Design review of the part built by this model. Coordinates are the model's own, in mm. Coordinates: 2 decimals unless noted, no trailing zeros. Loops run counter-clockwise (first coordinate to the right, second up) from the corner with the lowest first, then second, coordinate; pieces in that order, holes last. Notation, with made-up numbers: (87.25, -15) -> (105.25, -15) arc R27 cw to (105.25, 1) -> close; hole circle Ø1 at (15, 83). An arc over 180 degrees is marked (long way). Answer as a JSON object with one key per item and string values.
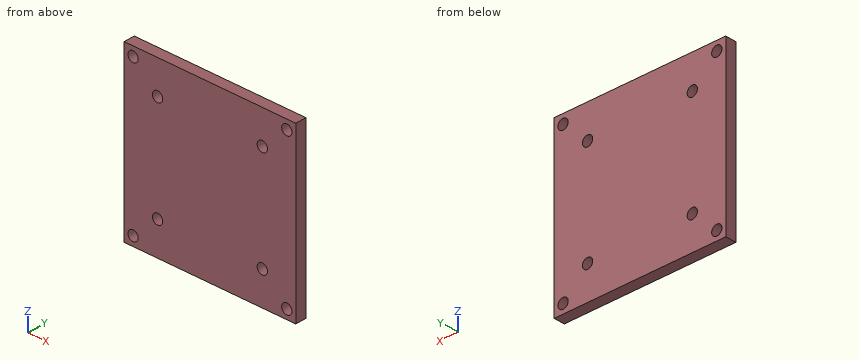
```python
from build123d import *

# Parameters (mm, degrees)
SKETCH1_W           = 50
SKETCH1_H           = 50
SKETCH1_R           = 1.5
BOSS_EXTRUDE1_DEPTH = 3.175


with BuildPart() as part:
    # Sketch1 → Boss-Extrude1 (new body)
    with BuildSketch(Plane(origin=(0, 0, 0), x_dir=(1, 0, 0), z_dir=(0, 1, 0))):
        Rectangle(SKETCH1_W, SKETCH1_H)
        with Locations((-22.4, 22.3)):
            Circle(SKETCH1_R, mode=Mode.SUBTRACT)
        with Locations((22.4, 22.3)):
            Circle(SKETCH1_R, mode=Mode.SUBTRACT)
        with Locations((22.4, -22.3)):
            Circle(SKETCH1_R, mode=Mode.SUBTRACT)
        with Locations((-22.4, -22.3)):
            Circle(SKETCH1_R, mode=Mode.SUBTRACT)
        with Locations((-15.25, 15.25)):
            Circle(SKETCH1_R, mode=Mode.SUBTRACT)
        with Locations((15.25, 15.25)):
            Circle(SKETCH1_R, mode=Mode.SUBTRACT)
        with Locations((15.25, -15.25)):
            Circle(SKETCH1_R, mode=Mode.SUBTRACT)
        with Locations((-15.25, -15.25)):
            Circle(SKETCH1_R, mode=Mode.SUBTRACT)
    extrude(amount=BOSS_EXTRUDE1_DEPTH)


solid = part.part
```
1) Add section A-A, the plane x = -22.4. Give the boundary of the cut face in (y, z) (3 decimals), and give its area (3 significant figures).
Completed:
{"outline": "(0, -25) -> (3.175, -25) -> (3.175, -23.8) -> (0, -23.8) -> close; (0, -20.8) -> (3.175, -20.8) -> (3.175, 20.8) -> (0, 20.8) -> close; (0, 23.8) -> (3.175, 23.8) -> (3.175, 25) -> (0, 25) -> close", "area": "140 mm²"}
2) Clearance check with flat-ended pins moving along their axes: pin 1 Ø5 at (x, z) = (22.4, 22.3) entering from +Y (3 decimals); pin 2 Ø2.5 at (x, z) = (22.4, -22.3) entering from +Y. State where each tip first meets the part, or that it passes through.
Completed:
{"pin 1": "y = 3.175", "pin 2": "through"}
3) Add section C-C, the plane z = -15.25. Give the boundary of the cut face in (x, y) (3 decimals), and give its area (3 significant figures).
Completed:
{"outline": "(-25, 0) -> (-16.75, 0) -> (-16.75, 3.175) -> (-25, 3.175) -> close; (-13.75, 0) -> (13.75, 0) -> (13.75, 3.175) -> (-13.75, 3.175) -> close; (16.75, 0) -> (25, 0) -> (25, 3.175) -> (16.75, 3.175) -> close", "area": "140 mm²"}
4) Add section B-B, the plane y = 1.9. Count the separate pieces of the cut face and the enclosed holes in it, and give its area (3 significant figures).
Completed:
{"separate pieces": "1", "enclosed holes": "8", "area": "2,440 mm²"}
5) Wall thickness on probe 1 along Z at (x, y) = (15.25, 1.55); probe 2 along X at (y, z) = (2.25, 22.3): over which ranges is each line inside the solid? List them lowest first.
Completed:
{"probe 1": "-25 to -16.75, -13.75 to 13.75, 16.75 to 25", "probe 2": "-25 to -23.9, -20.9 to 20.9, 23.9 to 25"}
